Geometry: final body of the model. Coordinates: model frame, mm. Face numbers are marked on the shaded views. A direction names the side the tool comes from. Give positions to 0.01 mm unless a question says otherwise; leave off trailing zeros. Write each loop counter-clockwise with the first axis right and the second up, starting at its lowest first coordinate (ties: lowest second). Pieces come first, ordered by that corner, then holes. Notation, with made-up numbers: M -29,-5 L -18,-5 A32 ccw -18,26 Z; hole C 83,67 d6. An arc over 180 degrees is marked long. Answer as a JSON object with one key per item and string values.
from build123d import *

# Parameters (mm, degrees)
F1_DEPTH      = 150
F1_DEPTH_BACK = 150
F0_W          = 49.6755242348
F0_H          = 124.2471858859
F2_DEPTH      = 120
F2_DEPTH_BACK = 120
F4_D          = 50
F4_DEPTH      = 62.124592943


with BuildPart() as f1:
    # F0 (on Front) → F1 (new body, two sides)
    with BuildSketch(Plane.XZ) as f1_sk:
        with BuildLine():
            Line((-39.2000116408, 62.123592943), (-70.0469091535, 62.123592943))
            ThreePointArc((-70.0469091535, 62.123592943), (0, 0.0945745131), (70.0469091535, 62.123592943))
            Line((70.0469091535, 62.123592943), (39.2000116408, 62.123592943))
            Line((39.2000116408, 62.123592943), (39.2000116408, 26.8699936569))
            Line((39.2000116408, 26.8699936569), (-39.2000116408, 26.8699936569))
            Line((-39.2000116408, 26.8699936569), (-39.2000116408, 62.123592943))
        make_face()
        with BuildLine():
            ThreePointArc((39.2000116408, 62.123592943), (0, 27.2705569476), (-39.2000116408, 62.123592943))
            Line((-39.2000116408, 62.123592943), (-39.2000116408, 26.8699936569))
            Line((-39.2000116408, 26.8699936569), (39.2000116408, 26.8699936569))
            Line((39.2000116408, 26.8699936569), (39.2000116408, 62.123592943))
        make_face()
    extrude(amount=F1_DEPTH)
    extrude(f1_sk.sketch, amount=-F1_DEPTH_BACK)

    # F0 (on Front) → F2 (join, two sides)
    with BuildSketch(Plane.XZ) as f2_sk:
        with Locations((-94.8846712708, 0)):
            Rectangle(F0_W, F0_H)
        with BuildLine():
            ThreePointArc((70.0469091535, 62.123592943), (0, 0.0945745131), (-70.0469091535, 62.123592943))
            Line((-70.0469091535, 62.123592943), (-70.0469091535, -62.123592943))
            Line((-70.0469091535, -62.123592943), (70.0469091535, -62.123592943))
            Line((70.0469091535, -62.123592943), (70.0469091535, 62.123592943))
        make_face()
        with Locations((94.8846712708, 0)):
            Rectangle(F0_W, F0_H)
    extrude(amount=F2_DEPTH)
    extrude(f2_sk.sketch, amount=-F2_DEPTH_BACK)

    # F4 (through all, one way)
    with BuildSketch(Plane.XY):
        with Locations((-84.6987441182, 0), (81.8660110235, 0)):
            Circle(F4_D / 2)
    extrude(amount=-F4_DEPTH, mode=Mode.SUBTRACT)


solid = f1.part
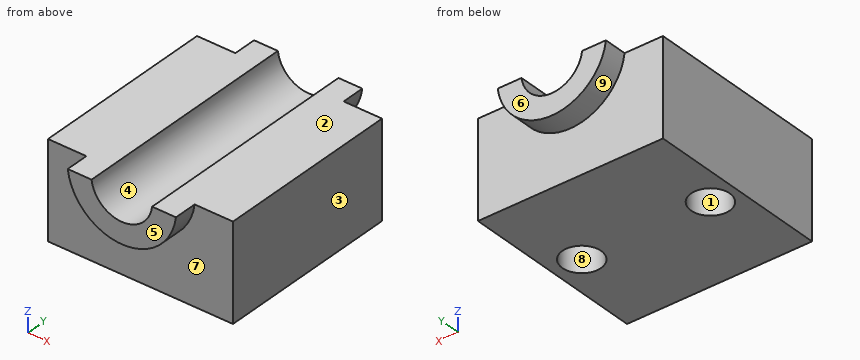
1) Cut plane A-A on z = -16.5. Return loops of the section in (x, y), and give its area (3 significant figures).
Geometry check:
{"outline": "M -119.72,-120 L 119.72,-120 L 119.72,120 L -119.72,120 Z; hole C -84.7,0 d50; hole C 81.87,0 d50", "area": "53,500 mm2"}
2) Line query: line 1 (X direction, y = -2.5, z = -49.5); line 2 (Y direction, x = 54, z = -26.5); line 3 (X direction, y = 87, z = 43). Output: solid intervals per line, ascending. Write a range as from..to.
Geometry check:
{"line 1": "x = -119.72..-109.57, -59.82..56.99, 106.74..119.72", "line 2": "y = -120..120", "line 3": "x = -119.72..-31.53, 31.53..119.72"}
3) Cut plane D-D on x = -19. Return loops of the section in (y, z).
Geometry check:
{"outline": "M -150,2.7 L -120,2.7 L -120,-62.12 L 120,-62.12 L 120,2.7 L 150,2.7 L 150,32.14 L -150,32.14 Z"}
4) Contact query for flat-ended pins moving along their axis: P1, Ø5, axis at x = -50.5, z = 14.5, coming from the +Y side; P2, Ø2, axis at x = 15, y = -108.5, coming from the +Z side. Output: stop coordinate, or through.
Geometry check:
{"P1": "stops at y = 120", "P2": "stops at z = 30.66"}
5) Cut plane C-C on z = 48.5. Return loops of the section in (x, y), and give its area (3 significant figures).
Geometry check:
{"outline": "M -119.72,-120 L -67,-120 L -67,-150 L -35,-150 L -35,150 L -67,150 L -67,120 L -119.72,120 Z; M 35,-150 L 67,-150 L 67,-120 L 119.72,-120 L 119.72,120 L 67,120 L 67,150 L 35,150 Z", "area": "44,500 mm2"}
6) Cut plane B-B on y = 0. Return loops of the section in (x, z), and give its area (3 significant figures).
Geometry check:
{"outline": "M -119.72,-62.12 L -109.7,-62.12 L -109.7,0 L -59.7,0 L -59.7,-62.12 L 56.87,-62.12 L 56.87,0 L 106.87,0 L 106.87,-62.12 L 119.72,-62.12 L 119.72,62.12 L 39.2,62.12 A39.47 cw -39.2,62.12 L -119.72,62.12 Z", "area": "21,500 mm2"}
7) Set-up query: the marked faces 5, 6, 7, 8 and 9. Return all of +Z, -Z, +X, -X, +Y, -Y with unobstructed straight access to the full face (end or side cutting, diameter ignored); none if empty.
Geometry check:
{"face 5": "+Z, -Z, +X, -X, -Y", "face 6": "+Z, -Z, +X, -X, +Y", "face 7": "-Z, -Y", "face 8": "-Z", "face 9": "-Z, +Y"}
8) Pull-direction query (X, two-part tool) for the marked faces 1, 2, 3 and 4; classes: pulls with the +X half, pulls with the -X half, needs draft (parallel to the pull), parting line crosses it, or undercut.
Geometry check:
{"face 1": "undercut", "face 2": "needs draft", "face 3": "pulls with the +X half", "face 4": "undercut"}
